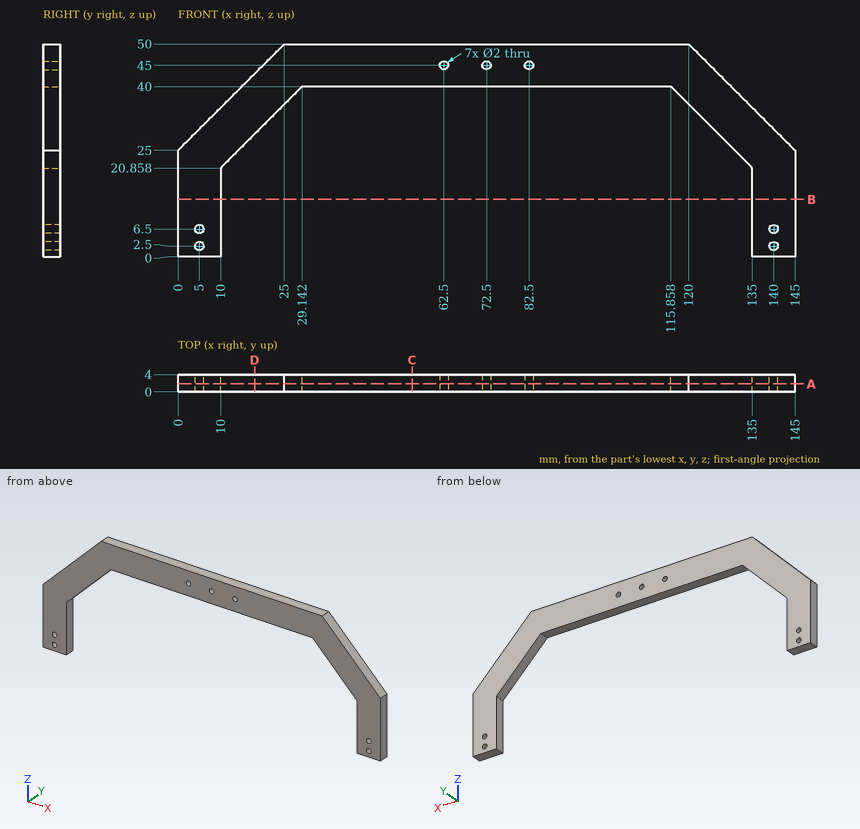
Input: dimensioned drawing with shaded views. Units: mm. Origin: part minimum x, y, z. Give positions to 0.01 mm unless a question says otherwise; leave off trailing zeros. Order: outer loops, then holes, each group sorted by start corner. A loop starts at its lowest first (then second) coordinate and runs counter-clockwise, first axis right, second up.
(1) Section query D-D (x = 18). Return the cut outline in (y, z), plus the area to 3 significant figures.
(2) Section query A-A (y = 1.85). Return the cut outline in (x, z).
(3) Contact query for flat-ended pins moving along their axis: P1, Ø1.8, axis at x = 140, z = 2.5, coming from the -Y side; P2, Ø2, axis at x = 55, y = 3, coming from the -Z side; P3, Ø1, axis at x = 17.5, y = 1.5, coming from the -Z side. Output: stop coordinate, or through.
(4) Section query C-C (x = 55). Return the cut outline in (y, z), plus the area to 3 significant figures.
(5) Section query B-B (z = 13.5). Return the cut outline in (x, y).
(6) Material intervals for line 1 along X through (y, z) = (0.9, 2.5); line 2 along X through (y, z) = (0.6, 4); line 3 along X through (y, z) = (2.4, 45), sorted ascending.
Outcome:
1. outline: (0, 28.86) - (4, 28.86) - (4, 43) - (0, 43) - close
1. area: 56.6 mm2
2. outline: (0, 0) - (10, 0) - (10, 20.86) - (29.14, 40) - (115.86, 40) - (135, 20.86) - (135, 0) - (145, 0) - (145, 25) - (120, 50) - (25, 50) - (0, 25) - close; hole circle Ø2 at (5, 2.5); hole circle Ø2 at (5, 6.5); hole circle Ø2 at (62.5, 45); hole circle Ø2 at (72.5, 45); hole circle Ø2 at (82.5, 45); hole circle Ø2 at (140, 2.5); hole circle Ø2 at (140, 6.5)
3. P1: passes through
3. P2: stops at z = 40
3. P3: stops at z = 27.86
4. outline: (0, 40) - (4, 40) - (4, 50) - (0, 50) - close
4. area: 40.0 mm2
5. outline: (0, 0) - (10, 0) - (10, 4) - (0, 4) - close; (135, 0) - (145, 0) - (145, 4) - (135, 4) - close
6. line 1: x = 0 to 4, 6 to 10, 135 to 139, 141 to 145
6. line 2: x = 0 to 10, 135 to 145
6. line 3: x = 20 to 61.5, 63.5 to 71.5, 73.5 to 81.5, 83.5 to 125
